The figure shows three views and two pictorial views of one solid part (mm, origin at its lowest corner). Answer the questions. Give positions to 0.01 mm unless a question says otherwise; leave off trailing zeros. Loops run counter-clockwise (first coordinate to the right, second up) from the corner with the lowest first, then second, coordinate; pieces in that order, holes last. Notation, with made-up numbers: M 76.5,9 L 118.5,9 A26 cw 118.5,27 Z; hole C 15.5,-28 d9. An arc over 180 degrees is marked long. One line per item, written item: value. Start each with the question number.
Q1. A cutting plane is placed at C-C, the plane x = 13.5. Determine the outline of the cut face in (y, z).
Q2. A cutting plane is placed at D-D, the plane y = 27.5. Determine the outline of the cut face in (x, z).
Q3. A cutting plane is placed at B-B, the plane y = 11.5. Determine the outline of the cut face in (x, z), and give its area (3 significant figures).
Q4. A cutting plane is placed at A-A, the plane z = 7.75. Determine the outline of the cut face in (x, y).
Q5. Consider L1, parallel to X at y = 14.25, z = 9.75; L2, parallel to X at y = 9, z = 7.5; L3, parallel to X at y = 21.75, z = 17.5. Determine where each line is inside the solid, lowest interval first.
Q6. Flat-ended cylindrical pins translate along their axes: pin 1 (15 mm diameter, centred on x = 159.5, y = 10.5, fed in from +Z); pin 2 (8 mm diameter, centred on y = 21.5, z = 17.5, fed in from -X); pin 3 (5 mm diameter, centred on y = 14.5, z = 13.5, fed in from +X). Find the tip coordinate at first contact, or state that the pin passes through.
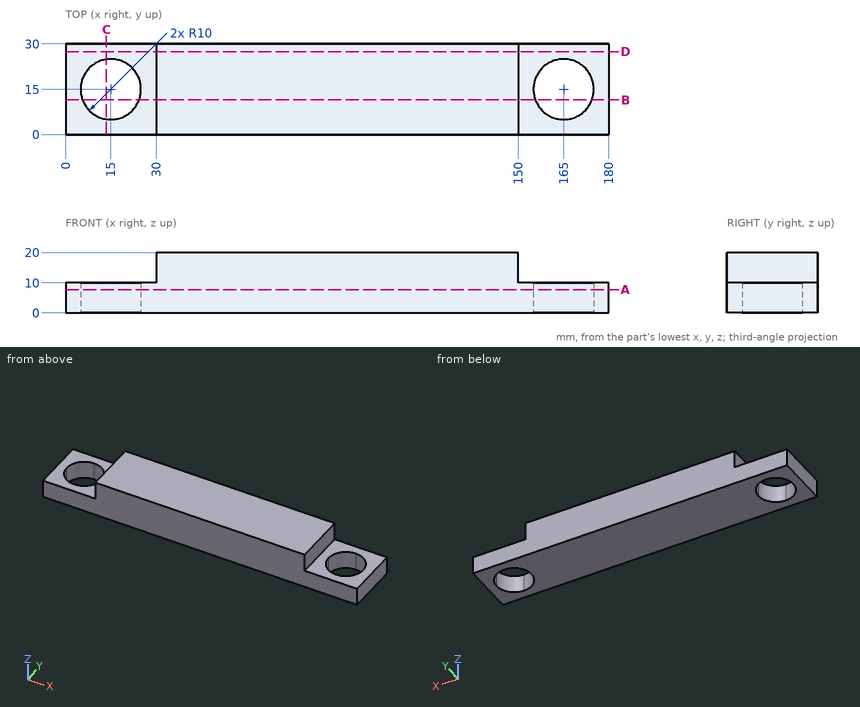
Answer block:
1. outline: M 0,0 L 5.11,0 L 5.11,10 L 0,10 Z; M 24.89,0 L 30,0 L 30,10 L 24.89,10 Z
2. outline: M 0,0 L 180,0 L 180,10 L 150,10 L 150,20 L 30,20 L 30,10 L 0,10 Z
3. outline: M 0,0 L 5.63,0 L 5.63,10 L 0,10 Z; M 24.37,0 L 155.63,0 L 155.63,10 L 150,10 L 150,20 L 30,20 L 30,10 L 24.37,10 Z; M 174.37,0 L 180,0 L 180,10 L 174.37,10 Z
3. area: 2,630 mm^2
4. outline: M 0,0 L 180,0 L 180,30 L 0,30 Z; hole M 5,15 A10 ccw 15,5 A10 ccw 25,15 A10 ccw 15,25 A10 ccw Z; hole M 155,15 A10 ccw 165,5 A10 ccw 175,15 A10 ccw 165,25 A10 ccw Z
5. L1: 0 to 5.03, 24.97 to 155.03, 174.97 to 180
5. L2: 0 to 7, 23 to 157, 173 to 180
5. L3: 30 to 150
6. pin 1: z = 10
6. pin 2: x = 30
6. pin 3: x = 150
